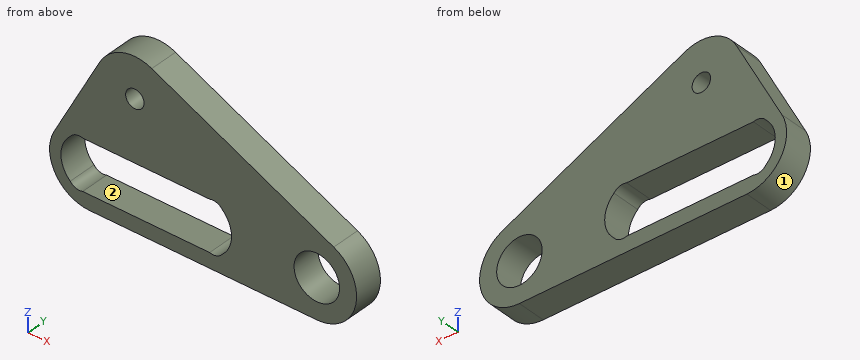
Autodesk Inventor part; units mm, degrees
ref_plane "YZ Plane" through (0, 0, 0) normal (1, 0, 0) x (0, 1, 0)
ref_plane "XZ Plane" through (0, 0, 0) normal (0, 1, 0) x (-1, 0, 0)
ref_plane "XY Plane" through (0, 0, 0) normal (0, 0, 1) x (1, 0, 0)
sketch "Sketch1" plane through (0, 0, 0) normal (0, 1, 0) x (-1, 0, 0)
  arc A0 (-2.971, 6.3382) -> (0, -7) centre (0, 0) ccw
  line L0 (0, 0) -> (40, 0) construction
  arc A1 (42.3749, -4.4) -> (42.3749, 4.4) centre (40, 0) ccw
  circle A2 centre (20, 0) radius 20 construction
  circle A3 centre (0, 0) radius 40 construction
  line L1 (42.3749, 4.4) -> (17.6251, 4.4)
  line L2 (0, 0) -> (10, -17.3205) construction
  line L3 (10, -17.3205) -> (20, -34.641) construction
  arc A4 (17.6251, 4.4) -> (17.6251, -4.4) centre (20, 0) ccw
  line L4 (42.3749, -4.4) -> (17.6251, -4.4)
  line L5 (30, 4.4) -> (30, -4.4) construction
  circle A5 centre (40, 0) radius 7 construction
  circle A6 centre (0, 0) radius 7 construction
  circle A7 centre (32, 15) radius 7 construction
  line L6 (-2.971, 6.3382) -> (29.029, 21.3382)
  line L7 (38.1765, 18.2941) -> (46.1765, 3.2941)
  line L8 (0, -7) -> (40, -7)
  arc A8 (40, -7) -> (46.1765, 3.2941) centre (40, 0) ccw
  arc A9 (38.1765, 18.2941) -> (29.029, 21.3382) centre (32, 15) ccw
  arc A10 (43.3651, 3.6981) -> (41.1611, 4.4) centre (41.768, 2.4943) ccw
  arc A11 (41.1611, -4.4) -> (43.3651, -3.6981) centre (41.768, -2.4943) ccw
  arc A12 (18.8389, 4.4) -> (16.6349, 3.6981) centre (18.232, 2.4943) ccw
  arc A13 (16.6349, -3.6981) -> (18.8389, -4.4) centre (18.232, -2.4943) ccw
  circle A14 centre (0, 0) radius 4 construction
  point P0 (16.6349, -3.6981)
  point P1 (16.6349, 3.6981)
  point P2 (18.8389, 4.4)
  point P3 (43.3651, -3.6981)
  point P4 (41.1611, -4.4)
  point P5 (18.8389, -4.4)
  dimension "d0" = 32
  dimension "d1" = 15
  dimension "d2" = 20
  dimension "d3" = 60
  dimension "d4" = 20
  dimension "d5" = 10
  dimension "d6" = 8.8
  dimension "d7" = 20
  dimension "d9" = 14
  dimension "d10" = 2
  dimension "d20" = 8
extrude "Extrusion1" add sketch "Sketch1" along normal blind 5
hole "Phi8.0-h7" at (0, 0, 0) direction (0, 1, 0) diameter 8 end through all
hole "M4" at (-32, 0, 15) direction (0, 1, 0) diameter 3.242 end through all
equation "\"d7\" = d4"
equation "\"d13\" = d20"
properties part number "ParallelLinksDriveFrame" material "Aluminum 7075"
Verification items for the finished model (mm, model axes). Face numbers are marked on the shaded views. A direction names the side the tool comes from. Coordinates: 2 decimals unless noted, no trailing zeros. Order: outer loops, then holes, each group sorted by start corner. A loop starts at its lowest first (then second) coordinate and runs counter-clockwise, first axis right, second up. Notation, with made-up numbers: (61, -23) - (100, -23) arc R20 ccw to (100, -16) - close; hole circle Ø6 at (69, -23.5). An arc over 180 degrees is marked (long way). Return JSON: item names as keys, results as strings.
(1) Go/stop test with flat-tipped pins: pin 1 (3 mm diameter, centred on y = 0.5, z = 12, fed in from -X); pin 2 (3 mm diameter, centred on y = 2.5, z = 12.5, fed in from +X); pin 3 (3 mm diameter, centred on x = -30, y = 1.5, fed in from +Z); pin 4 (5 mm diameter, centred on x = 0, z = 0, fed in from +Y). Record where each tip stops, or that it passes through.
Filled sheet:
{"pin 1": "stops at x = -42.33", "pin 2": "stops at x = -6.97", "pin 3": "stops at z = 21.98", "pin 4": "passes through"}
(2) Section check A-A, the plane z = 0. Record the cut outline in (x, y), and give its area (3 significant figures).
Filled sheet:
{"outline": "(-47, 0) - (-45, 0) - (-45, 5) - (-47, 5) - close; (-15, 0) - (-4, 0) - (-4, 5) - (-15, 5) - close; (4, 0) - (7, 0) - (7, 5) - (4, 5) - close", "area": "80.0 mm^2"}
(3) Thickness scan on line 1 along X through (y, z) = (1.9, 0); line 2 along Z through (x, y) = (-32, 3.6); line 3 along X through (y, z) = (2.7, 2.5). Record the ranges inside material, lowest first.
Filled sheet:
{"line 1": "x = -47 to -45, -15 to -4, 4 to 7", "line 2": "z = -7 to -4.4, 4.4 to 13.38, 16.62 to 22", "line 3": "x = -46.54 to -44.33, -15.67 to -3.12, 3.12 to 6.54"}
(4) Section check D-D, the plane y = 2.65. Record the cut outline in (x, z), and give its area (3 significant figures).
Filled sheet:
{"outline": "(-46.18, 3.29) arc R7 ccw to (-40, -7) - (0, -7) arc R7 ccw to (2.97, 6.34) - (-29.03, 21.34) arc R7 ccw to (-38.18, 18.29) - close; hole (-43.37, -3.7) arc R2 ccw to (-41.16, -4.4) - (-18.84, -4.4) arc R2 ccw to (-16.63, -3.7) arc R5 ccw to (-16.63, 3.7) arc R2 ccw to (-18.84, 4.4) - (-41.16, 4.4) arc R2 ccw to (-43.37, 3.7) arc R5 ccw to start; hole circle Ø3.24 at (-32, 15); hole circle Ø8 at (0, 0)", "area": "791 mm^2"}
(5) Section check C-C, the plane x = -2.5. Record the cut outline in (y, z).
Filled sheet:
{"outline": "(0, -7) - (5, -7) - (5, -3.12) - (0, -3.12) - close; (0, 3.12) - (5, 3.12) - (5, 8.9) - (0, 8.9) - close"}
(6) Section check B-B, the plane x = -32. Record the cut outline in (y, z), and give its area (3 significant figures).
Filled sheet:
{"outline": "(0, -7) - (5, -7) - (5, -4.4) - (0, -4.4) - close; (0, 4.4) - (5, 4.4) - (5, 13.38) - (0, 13.38) - close; (0, 16.62) - (5, 16.62) - (5, 22) - (0, 22) - close", "area": "84.8 mm^2"}
(7) Access from +Z, -Z, +X, -X, +Y, -Y to the whole of each face (thin tool, end or side, straight path). Record for the marked faces 1 and 2.
Filled sheet:
{"face 1": "-X, +Y, -Y", "face 2": "+Y, -Y"}
